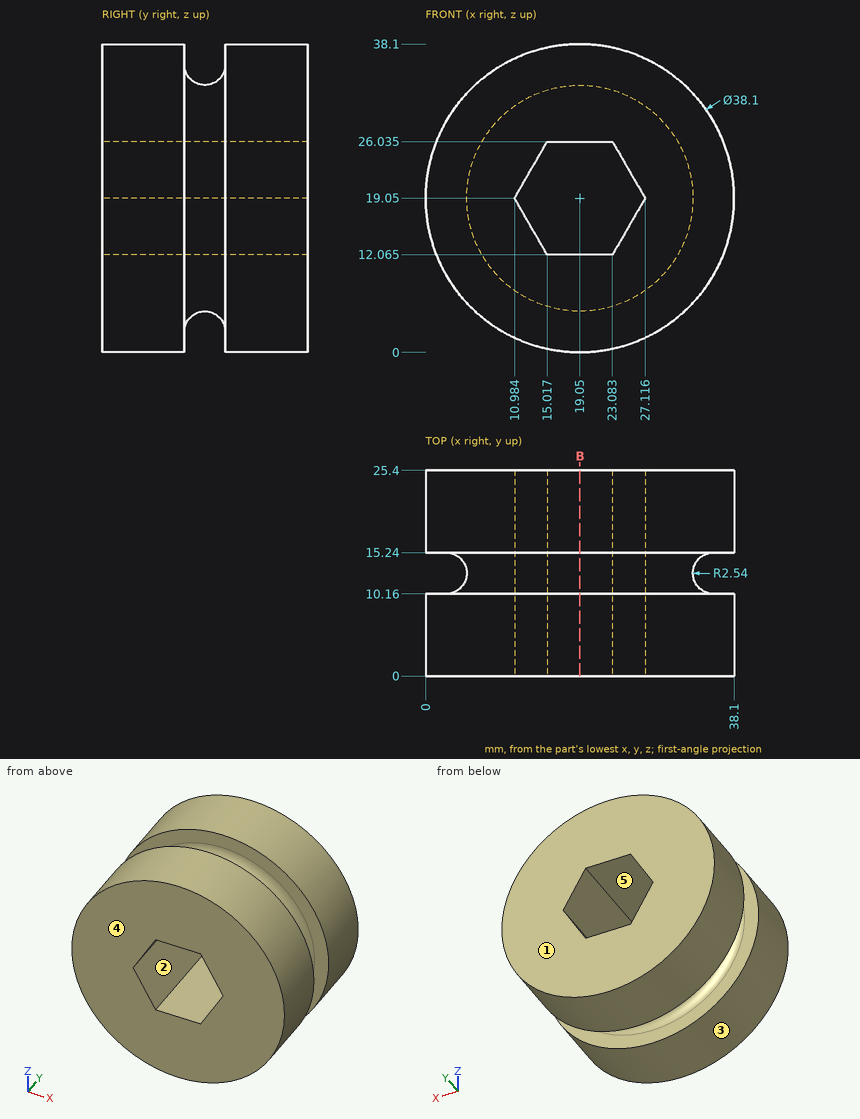
Design review of the part shown in the three views and the two pictorial views. Dimensions are in mm from the part's minimum x, y and z. A direction names the side the tool comes from. Round coordinates to 2 decimals unless told otherwise and drop trailing zeros. Order: outer loops, then holes, each group sorted by start corner. A loop starts at its lowest first (then second) coordinate and runs counter-clockwise, first axis right, second up.
(1) Tool access review of the marked faces 4 and 5: name each direction out of +Z, -Z, +X, -X, +Y, -Y from which nothing blocks a thin tool from reaching the whole face with its end or side.
Working result:
face 4: +Z, -Z, +X, -X, -Y
face 5: +Y, -Y
(2) For P1, Ø10, axis at y = 12, z = 10, coming from the -X side (1 decimal); P2, Ø1, axis at y = 16, z = 7.5, coming from the -X side; P3, Ø1, axis at x = 31, y = 16, coming from the +Z side (1 decimal), all flat-tipped, find the tip position at first contact; note any pin that passes through.
Working result:
P1: stops at x = 0.5
P2: stops at x = 3.53
P3: stops at z = 34.3
(3) Take a section at B-B, the plane x = 19.05. State the section outline as (y, z) points (1 decimal), plus the area to 3 significant figures.
Working result:
outline: (0, 0) - (10.2, 0) - (10.2, 2.5) arc R2.5 cw to (15.2, 2.5) - (15.2, 0) - (25.4, 0) - (25.4, 12.1) - (0, 12.1) - close; (0, 26) - (25.4, 26) - (25.4, 38.1) - (15.2, 38.1) - (15.2, 35.6) arc R2.5 cw to (10.2, 35.6) - (10.2, 38.1) - (0, 38.1) - close
area: 567 mm2
(4) Wall thickness on L1, parallel to Y at x = 34, z = 29.5; L2, parallel to X at y = 21.75, z = 13 (1 decimal); L3, parallel to X at y = 16, z = 23 (1 decimal): over which ranges is each line inside the solid? List them lowest first.
Working result:
L1: y = 0 to 10.16, 15.24 to 25.4
L2: x = 1 to 14.5, 23.6 to 37.1
L3: x = 0.4 to 13.3, 24.8 to 37.7
(5) Mouldability with a two-part tool opening along X and no side actions: class the marked faces 1, 2 and 3 as released by +X, released by -X, zero draft, split by the parting line, or undercut.
Working result:
face 1: zero draft
face 2: undercut
face 3: split by the parting line
